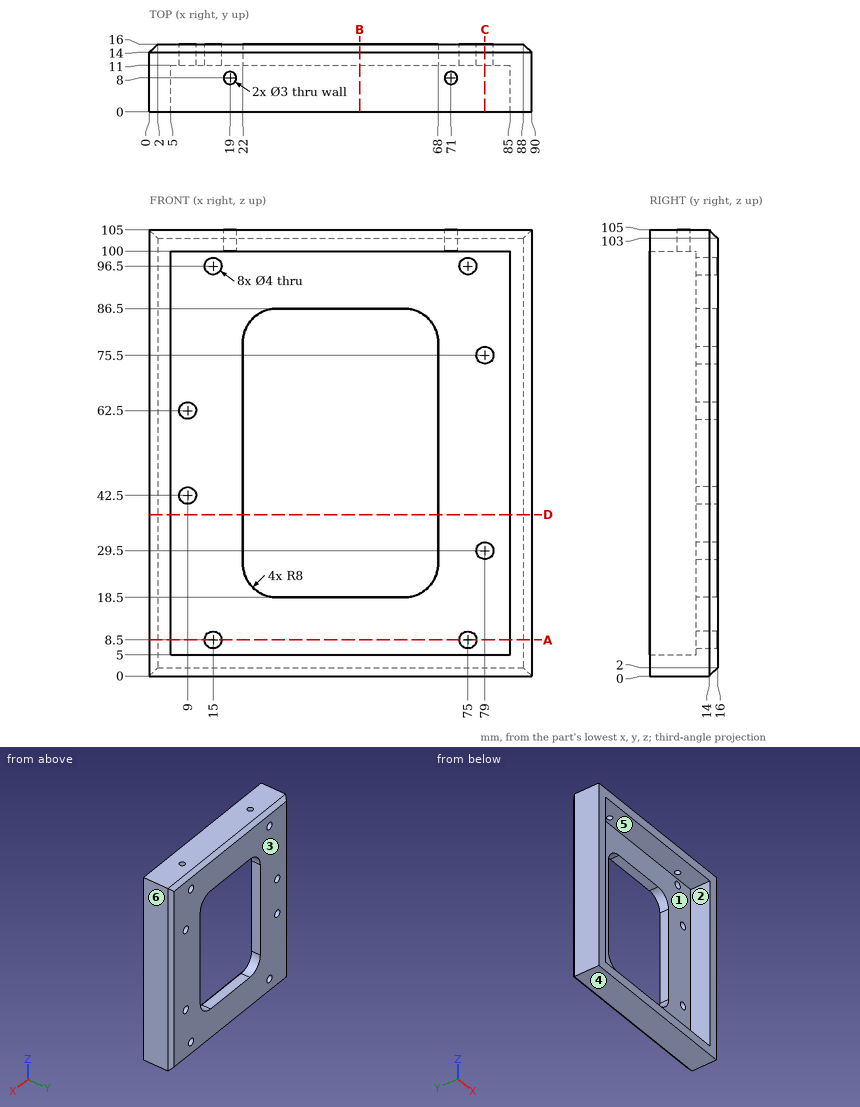
Check sheet for the drawn part. Datum: minimum x, y, z corner. Units: mm. A direction names the side the tool comes from. Coordinates: 2 decimals unless noted, no trailing zeros. Order: outer loops, then holes, each group sorted by start corner. A loop starts at its lowest first (then second) coordinate and runs counter-clockwise, first axis right, second up. Notation, with made-up numbers: (7, 60.25) -> (38, 60.25) arc R24 cw to (38, 71.25) -> close; hole circle Ø7 at (48.25, 83). An arc over 180 degrees is marked (long way). Use a Markdown table: item, result. Add a question column.
1. Cross-section at C-C (x = 79). Enter the section's corners in (y, z), and give its area (3 significant figures).
2. Cross-section at B-B (x = 49.5). Enter the section's corners in (y, z).
3. Mould release check, pull along Z, two halves, no side actions. Record for the marked faces 1, 2, 3 and 4: pulls with the +Z half, pulls with the -Z half, needs draft (parallel to the pull), parting line crosses it, or undercut.
4. Cross-section at D-D (z = 38). Enter the section's corners in (x, y).
5. Go/stop test with a flat-tipped pin: pin 1 Ø6 at (x, z) = (72, 20) entering from -Y. Record where the tip stops, or that it passes through.
6. Cross-section at A-A (z = 8.5). Enter the section's corners in (x, y), and give its area (3 significant figures).
7. Material ranges on L1, parallel to X at y = 12.2, z = 62.5; L2, parallel to Z at x = 32.5, y = 6.75; L3, parallel to X at y = 7.5, z = 67, recorded low to high.
8. Set-up check for the marked faces 5 and 6: record each of +Z, -Z, +X, -X, +Y, -Y from which the full face is reachable in a straight line by a thin tool's end or side.
Filled sheet:
| question | item | result |
|---|---|---|
| 1 | outline | (0, 0) -> (14, 0) -> (16, 2) -> (16, 27.5) -> (11, 27.5) -> (11, 5) -> (0, 5) -> close; (0, 100) -> (11, 100) -> (11, 77.5) -> (16, 77.5) -> (16, 103) -> (14, 105) -> (0, 105) -> close; (11, 31.5) -> (16, 31.5) -> (16, 73.5) -> (11, 73.5) -> close |
| 1 | area | 591 mm2 |
| 2 | outline | (0, 0) -> (14, 0) -> (16, 2) -> (16, 18.5) -> (11, 18.5) -> (11, 5) -> (0, 5) -> close; (0, 100) -> (11, 100) -> (11, 86.5) -> (16, 86.5) -> (16, 103) -> (14, 105) -> (0, 105) -> close |
| 3 | face 1 | undercut |
| 3 | face 2 | undercut |
| 3 | face 3 | needs draft |
| 3 | face 4 | pulls with the -Z half |
| 4 | outline | (0, 0) -> (5, 0) -> (5, 11) -> (22, 11) -> (22, 16) -> (2, 16) -> (0, 14) -> close; (68, 11) -> (85, 11) -> (85, 0) -> (90, 0) -> (90, 14) -> (88, 16) -> (68, 16) -> close |
| 5 | pin 1 | y = 11 |
| 6 | outline | (0, 0) -> (5, 0) -> (5, 11) -> (13, 11) -> (13, 16) -> (2, 16) -> (0, 14) -> close; (17, 11) -> (73, 11) -> (73, 16) -> (17, 16) -> close; (77, 11) -> (85, 11) -> (85, 0) -> (90, 0) -> (90, 14) -> (88, 16) -> (77, 16) -> close |
| 6 | area | 516 mm2 |
| 7 | L1 | 0 to 7, 11 to 22, 68 to 90 |
| 7 | L2 | 0 to 5, 100 to 105 |
| 7 | L3 | 0 to 5, 85 to 90 |
| 8 | face 5 | -Y |
| 8 | face 6 | +Z, -Z, +X, +Y, -Y |
